Work out the finished part from the listing and answer in its coordinate system (mm). A direction names the side the tool comes from. Coordinates: 2 decimals unless noted, no trailing zeros. Write each loop counter-clockwise with the first axis right and the second up, starting at its lowest first coordinate (ties: lowest second). Pieces come first, ordered by that corner, then holes. Notation, with made-up numbers: (-27, 61) -> (-5, 61) arc R13 cw to (-5, 78) -> close; hole circle Ø3 at (85, 89.25). An arc over 180 degrees is marked (long way). Write each question's results on one line, items separated by ' | '. Start each with the question number.
from build123d import *

# Parameters (mm, degrees)
BOSS_EXTRUDE1_DEPTH = 8
SKETCH2_W           = 150
SKETCH2_H           = 8
BOSS_EXTRUDE2_DEPTH = 50


with BuildPart() as part:
    # Sketch1 → Boss-Extrude1 (new body)
    with BuildSketch(Plane.XY):
        Polygon((-15, 15), (-15, 60), (15, 60), (15, 15), (75, 15), (75, -35), (-75, -35), (-75, 15), align=None)
        with BuildLine():
            Line((-2.5, 2.5), (-50, 2.5))
            ThreePointArc((-50, 2.5), (-52.5, 0), (-50, -2.5))
            Line((-50, -2.5), (50, -2.5))
            ThreePointArc((50, -2.5), (52.5, 0), (50, 2.5))
            Line((50, 2.5), (2.5, 2.5))
            Line((2.5, 2.5), (2.5, 50))
            ThreePointArc((2.5, 50), (0, 52.5), (-2.5, 50))
            Line((-2.5, 50), (-2.5, 2.5))
        make_face(mode=Mode.SUBTRACT)
    extrude(amount=-BOSS_EXTRUDE1_DEPTH)

    # Sketch2 → Boss-Extrude2 (add)
    with BuildSketch(Plane.XY):
        with Locations((0, -31)):
            Rectangle(SKETCH2_W, SKETCH2_H)
    extrude(amount=BOSS_EXTRUDE2_DEPTH)


solid = part.part
1. Find section C-C on y = 38. Give the vertices of the cut face in (x, z).
2. For faces 5 (the face through (-15, 37, -4)), 6 (the face through (-2.5, 27, -4)), 7 (the face through (15, 38, -4)), determine the directions among +Z, -Z, +X, -X, +Y, -Y from which every point of the face is accessible in a straight line to the end or side of a thin tool.
3. Find section B-B on x = -21. Give the vertices of the cut face in (y, z).
4. Find section D-D on x = 55. Give the vertices of the cut face in (y, z), and give its area (3 significant figures).
5. Find the intervals of material crossed by L1, parallel to Y at x = 11.5, z = -5; L2, parallel to X at y = 5, z = -2; L3, parallel to Y at x = -26, z = -2, in increasing order.
6. Determine the mould class of faces 1 (the face through (75, -29, 8)), 2 (the face through (-1, -2.5, -4)), 3 (the face through (-45, 15, -4)), 4 (the face through (52.5, -0.1, -3.9)) for opening direction X: pulls with the +X half, pulls with the -X half, needs draft (parallel to the pull), parting line crosses it, or undercut.
7. Given pin 1 Ø6.5 at (x, z) = (49.5, -2.5) entering from +Y; pin 2 Ø4 at (y, z) = (41, -3) entering from -X; pin 3 Ø4 at (y, z) = (31.5, -2.5) entering from +X, each flat-ended and moving along its own axis, determine where each tip first touches the part or whether it passes through.
8. Find section A-A on y = 0. Give the vertices of the cut face in (x, z).
Ans:
1) outline: (-15, -8) -> (-2.5, -8) -> (-2.5, 0) -> (-15, 0) -> close; (2.5, -8) -> (15, -8) -> (15, 0) -> (2.5, 0) -> close
2) face 5: +Z, -Z, -X, +Y | face 6: +Z, -Z | face 7: +Z, -Z, +X, +Y
3) outline: (-35, -8) -> (-2.5, -8) -> (-2.5, 0) -> (-27, 0) -> (-27, 50) -> (-35, 50) -> close; (2.5, -8) -> (15, -8) -> (15, 0) -> (2.5, 0) -> close
4) outline: (-35, -8) -> (15, -8) -> (15, 0) -> (-27, 0) -> (-27, 50) -> (-35, 50) -> close | area: 800 mm²
5) L1: y = -35 to -2.5, 2.5 to 60 | L2: x = -75 to -2.5, 2.5 to 75 | L3: y = -35 to -2.5, 2.5 to 15
6) face 1: pulls with the +X half | face 2: undercut | face 3: needs draft | face 4: undercut
7) pin 1: stops at y = 15 | pin 2: stops at x = -15 | pin 3: stops at x = 15
8) outline: (-75, -8) -> (-52.5, -8) -> (-52.5, 0) -> (-75, 0) -> close; (52.5, -8) -> (75, -8) -> (75, 0) -> (52.5, 0) -> close
